Input: part model. Units: mm. Frame: model coordinates. A direction names the side the tool comes from. Coordinates: 2 decimals unless noted, no trailing zeros. Loops run counter-clockwise (first coordinate to the right, second up) from the corner with the lowest first, then second, coordinate; pieces in that order, holes last.
Item 1: Pull-direction query (Y, two-part tool) for faces 3 (the flat face through (0, 0, 2)), 4 (the flat face through (-0.04, 7.33, 3.5)), 5 (the flat face through (-2.625, 4, 2)); classes: released by +Y, released by -Y, zero draft, split by the parting line, or undercut.
Item 2: Contact query for flat-ended pins moving along their axis: P1, Ø2, axis at y = 3.5, z = 2.5, coming from the -X side; P2, Ø2, axis at x = -3, y = 4.5, coming from the +Z side. Output: stop coordinate, or through.
Item 3: Section A-A on y = 4. Return loops of the section in (x, z) (3 decimals).
Item 4: Section D-D on y = 1.75. Return loops of the section in (x, z) (3 decimals), and give its area (3 significant figures).
Item 5: Ray query, line 1 along X through (y, z) = (4, 0.6); line 2 along Y through (x, z) = (0, 0.5); line 3 along Z through (x, y) = (2.25, 3.5). Return the intervals inside material, ascending.
Item 6: Section B-B on z = 2.9. Return loops of the section in (x, y) (3 decimals), and give its area (3 significant figures).
Item 7: Section C-C on x = 0.75. Return loops of the section in (y, z).
Item 8: Reachability of faces 1 (the flat face through (0, 6, 0)), 2 (the flat face through (-1.331, 1.605, 2.268)) from +Z, -Z, +X, -X, +Y, -Y: full face, straight path, thin tool, end or side. Return the list, or none.
Autodesk Fusion 360 part; units mm, degrees
sketch "Sketch1" plane through (0, 0, 0) normal (0, 1, 0) x (1, 0, 0)
  line L0 (0, 0) -> (5.5, 0)
  line L1 (0, -3.5) -> (2.625, -3.5)
  line L2 (2.625, -3.5) -> (5.5, 0)
  line L3 (0, -1.75) -> (0, -22.5)
  line L4 (0, -3.5) -> (-2.625, -3.5)
  line L5 (-2.625, -3.5) -> (-5.5, 0)
  line L6 (0, 0) -> (-5.5, 0)
  line L7 (-4.5, -1.2174) -> (-4.5, 0)
  line L8 (4.5, -1.2174) -> (4.5, 0)
  dimension "d1" = 5.5
  dimension "d2" = 2.625
  dimension "d3" = 3.5
  dimension "d16" = 4.5
extrude "Extrude1" add sketch "Sketch1" along normal blind 8 contours L0 L1 L2 L4 L5 L6 L7 L8
sketch "Sketch2" plane through (0, 0, 3.5) normal (0, 0, 1) x (-1, 0, 0)
  line L0 (2.625, 0) -> (-2.625, 0)
  line L1 (-2.625, 0) -> (-2.625, -8)
  line L2 (-2.625, -8) -> (2.625, -8)
  line L3 (2.625, -8) -> (2.625, 0)
  line L4 (0, -8) -> (0, 0) construction
  line L5 (2.74, -2.4181) -> (0, -0.8361)
  line L6 (0, -0.8361) -> (-2.74, -2.4181)
  line L7 (-2.74, -2.4181) -> (-2.74, -5.5819)
  line L8 (-2.74, -5.5819) -> (0, -7.1639)
  line L9 (0, -7.1639) -> (2.74, -5.5819)
  line L10 (2.74, -5.5819) -> (2.74, -2.4181)
  line L11 (2.72, 25.0704) -> (0, 26.6408)
  line L12 (0, 26.6408) -> (-2.72, 25.0704)
  line L13 (-2.72, 25.0704) -> (-2.72, 21.9296)
  line L14 (-2.72, 21.9296) -> (0, 20.3592)
  line L15 (0, 20.3592) -> (2.72, 21.9296)
  line L16 (2.72, 21.9296) -> (2.72, 25.0704)
  point P0 (0, -4)
  dimension "d6" = 2.74
  dimension "d9" = 4
extrude "Extrude2" cut sketch "Sketch2" against normal blind 2.5 contours L1 L3 L5 L6 L8 L9 | L11 L12 L13 L14 L15 L16
hole "Hole1" at (0, 4, 3.5) direction (0, 0, -1) diameter 3.4 depth 16 tip angle 118
equation "d2 = ( 5.25 / 2 ) * 1 mm"
equation "d6 = ( 5.48 / 2 ) * 1 mm"
Results found:
1. face 3: released by -Y
1. face 4: zero draft
1. face 5: undercut
2. P1: stops at x = -4.27
2. P2: stops at z = 3.5
3. outline: (-4.5, 0) - (-1.7, 0) - (-1.7, 1) - (-2.625, 1) - (-2.625, 3.5) - (-4.5, 1.217) - close; (1.7, 0) - (4.5, 0) - (4.5, 1.217) - (2.625, 3.5) - (2.625, 1) - (1.7, 1) - close
4. outline: (-4.5, 0) - (4.5, 0) - (4.5, 1.217) - (2.625, 3.5) - (1.583, 3.5) - (1.583, 1) - (-1.583, 1) - (-1.583, 3.5) - (-2.625, 3.5) - (-4.5, 1.217) - close
4. area: 19.3 mm2
5. line 1: x = -4.5 to -1.7, 1.7 to 4.5
5. line 2: y = 0 to 2.3, 5.7 to 8
5. line 3: z = 0 to 1
6. outline: (-3.118, 0) - (3.118, 0) - (3.118, 8) - (-3.118, 8) - close; hole (-2.625, 2.352) - (0, 0.836) - (2.625, 2.352) - (2.625, 5.648) - (0, 7.164) - (-2.625, 5.648) - close
6. area: 24.6 mm2
7. outline: (0, 0) - (2.47, 0) - (2.47, 1) - (1.27, 1) - (1.27, 3.5) - (0, 3.5) - close; (5.53, 0) - (8, 0) - (8, 3.5) - (6.73, 3.5) - (6.73, 1) - (5.53, 1) - close
8. face 1: -Z, +X, -X, +Y, -Y
8. face 2: +Z
